```python
from build123d import *

# Parameters (mm, degrees)
SKETCH_1_R          = 50
EXTRUDE_1_DEPTH     = 20
SKETCH_2_R          = 5.25
CUT_EXTRUDE_1_DEPTH = 20
CUT_EXTRUDE_2_DEPTH = 20
SKETCH_4_R          = 50
SKETCH_4_R_2        = 5.25
EXTRUDE_2_DEPTH     = 20


with BuildPart() as part:
    # 草图1 → 凸台-拉伸1 (new body)
    with BuildSketch(Plane(origin=(0, 0, 0), x_dir=(1, 0, 0), z_dir=(0, 1, 0))):
        with Locations(Location((0, 0, 0), (0, 0, 270))):
            Circle(SKETCH_1_R)
    extrude(amount=EXTRUDE_1_DEPTH)

    # 草图2 → 切除-拉伸1 (cut)
    with BuildSketch(Plane(origin=(0, 20, 0), x_dir=(1, 0, 0), z_dir=(0, 1, 0))):
        with Locations(Location((0, 0, 0), (0, 0, 270))):
            Circle(SKETCH_2_R)
    extrude(amount=-CUT_EXTRUDE_1_DEPTH, mode=Mode.SUBTRACT)

    # 草图3 → 切除-拉伸2 (cut)
    with BuildSketch(Plane(origin=(0, 20, 0), x_dir=(1, 0, 0), z_dir=(0, 1, 0))):
        with BuildLine():
            ThreePointArc((42.5, 0), (35, 7.5), (27.5, 0))
            ThreePointArc((27.5, 0), (25.406687144, -10.52379439), (19.445436483, -19.445436483))
            ThreePointArc((19.445436483, -19.445436483), (19.445436477, -30.052038195), (30.052038189, -30.052038212))
            ThreePointArc((30.052038189, -30.052038212), (39.264880129, -16.264045883), (42.5, 0))
        make_face()
        with BuildLine():
            ThreePointArc((2e-09, 27.5), (10.523794391, 25.406687144), (19.445436483, 19.445436483))
            ThreePointArc((19.445436483, 19.445436483), (30.0520382, 19.445436483), (30.0520382, 30.0520382))
            ThreePointArc((30.0520382, 30.0520382), (16.264045902, 39.264880121), (5.8e-08, 42.5))
            ThreePointArc((5.8e-08, 42.5), (-7.5, 35.000000028), (2e-09, 27.5))
        make_face()
        with BuildLine():
            ThreePointArc((-30.0520382, -30.0520382), (-16.264045799, -39.264880163), (1.65e-07, -42.5))
            ThreePointArc((1.65e-07, -42.5), (7.5, -34.999999948), (6.1e-08, -27.5))
            ThreePointArc((6.1e-08, -27.5), (-10.523794348, -25.406687162), (-19.44543646, -19.445436505))
            ThreePointArc((-19.44543646, -19.445436505), (-30.052038189, -19.445436472), (-30.0520382, -30.0520382))
        make_face()
        with BuildLine():
            ThreePointArc((-27.5, 0), (-25.406687154, 10.523794365), (-19.445436521, 19.445436445))
            ThreePointArc((-19.445436521, 19.445436445), (-19.445436492, 30.05203821), (-30.052038258, 30.052038143))
            ThreePointArc((-30.052038258, 30.052038143), (-39.264880164, 16.264045797), (-42.5, -8.9e-08))
            ThreePointArc((-42.5, -8.9e-08), (-34.999999956, -7.5), (-27.5, 0))
        make_face()
    extrude(amount=-CUT_EXTRUDE_2_DEPTH, mode=Mode.SUBTRACT)

    # 草图4 → 凸台-拉伸2 (add)
    # profile 1 of 6: a face of its own
    with BuildSketch(Plane.XZ):
        with Locations(Location((0, 0, 0), (0, 0, 270))):
            Circle(SKETCH_4_R)
        with BuildLine():
            ThreePointArc((30.0520382, 30.0520382), (39.264880132, 16.264045876), (42.5, 0))
            ThreePointArc((42.5, 0), (39.264880132, -16.264045876), (30.0520382, -30.0520382))
            ThreePointArc((30.0520382, -30.0520382), (16.264045876, -39.264880132), (0, -42.5))
            ThreePointArc((0, -42.5), (-16.264045876, -39.264880132), (-30.0520382, -30.0520382))
            ThreePointArc((-30.0520382, -30.0520382), (-39.264880132, -16.264045876), (-42.5, 0))
            ThreePointArc((-42.5, 0), (-39.264880132, 16.264045876), (-30.0520382, 30.0520382))
            ThreePointArc((-30.0520382, 30.0520382), (-16.264045876, 39.264880132), (0, 42.5))
            ThreePointArc((0, 42.5), (16.264045876, 39.264880132), (30.0520382, 30.0520382))
        make_face(mode=Mode.SUBTRACT)
    # profile 2 of 6: a face of its own
    with BuildSketch(Plane.XZ):
        with BuildLine():
            ThreePointArc((0, -42.5), (-7.5, -35), (0, -27.5))
            ThreePointArc((0, -27.5), (-10.52379439, -25.406687144), (-19.445436483, -19.445436483))
            ThreePointArc((-19.445436483, -19.445436483), (-19.445436483, -30.0520382), (-30.0520382, -30.0520382))
            ThreePointArc((-30.0520382, -30.0520382), (-16.264045876, -39.264880132), (0, -42.5))
        make_face()
    # profile 3 of 6: a face of its own
    with BuildSketch(Plane.XZ):
        with BuildLine():
            ThreePointArc((-27.5, 0), (-25.406687144, 10.52379439), (-19.445436483, 19.445436483))
            ThreePointArc((-19.445436483, 19.445436483), (-30.0520382, 19.445436483), (-30.0520382, 30.0520382))
            ThreePointArc((-30.0520382, 30.0520382), (-39.264880132, 16.264045876), (-42.5, 0))
            ThreePointArc((-42.5, 0), (-35, 7.5), (-27.5, 0))
        make_face()
    # profile 4 of 6: a face of its own
    with BuildSketch(Plane.XZ):
        with BuildLine():
            ThreePointArc((0, 27.5), (10.52379439, 25.406687144), (19.445436483, 19.445436483))
            ThreePointArc((19.445436483, 19.445436483), (19.445436483, 30.0520382), (30.0520382, 30.0520382))
            ThreePointArc((30.0520382, 30.0520382), (16.264045876, 39.264880132), (0, 42.5))
            ThreePointArc((0, 42.5), (7.5, 35), (0, 27.5))
        make_face()
    # profile 5 of 6: a face of its own
    with BuildSketch(Plane.XZ):
        with BuildLine():
            ThreePointArc((19.445436483, -19.445436483), (25.406687144, -10.52379439), (27.5, 0))
            ThreePointArc((27.5, 0), (25.406687144, 10.52379439), (19.445436483, 19.445436483))
            ThreePointArc((19.445436483, 19.445436483), (10.52379439, 25.406687144), (0, 27.5))
            ThreePointArc((0, 27.5), (-10.52379439, 25.406687144), (-19.445436483, 19.445436483))
            ThreePointArc((-19.445436483, 19.445436483), (-25.406687144, 10.52379439), (-27.5, 0))
            ThreePointArc((-27.5, 0), (-25.406687144, -10.52379439), (-19.445436483, -19.445436483))
            ThreePointArc((-19.445436483, -19.445436483), (-10.52379439, -25.406687144), (0, -27.5))
            ThreePointArc((0, -27.5), (10.52379439, -25.406687144), (19.445436483, -19.445436483))
        make_face()
        with Locations(Location((0, 0, 0), (0, 0, 90))):
            Circle(SKETCH_4_R_2, mode=Mode.SUBTRACT)
    # profile 6 of 6: a face of its own
    with BuildSketch(Plane.XZ):
        with BuildLine():
            ThreePointArc((42.5, 0), (35, -7.5), (27.5, 0))
            ThreePointArc((27.5, 0), (25.406687144, -10.52379439), (19.445436483, -19.445436483))
            ThreePointArc((19.445436483, -19.445436483), (30.0520382, -19.445436483), (30.0520382, -30.0520382))
            ThreePointArc((30.0520382, -30.0520382), (39.264880132, -16.264045876), (42.5, 0))
        make_face()
    extrude(amount=EXTRUDE_2_DEPTH)


solid = part.part
```
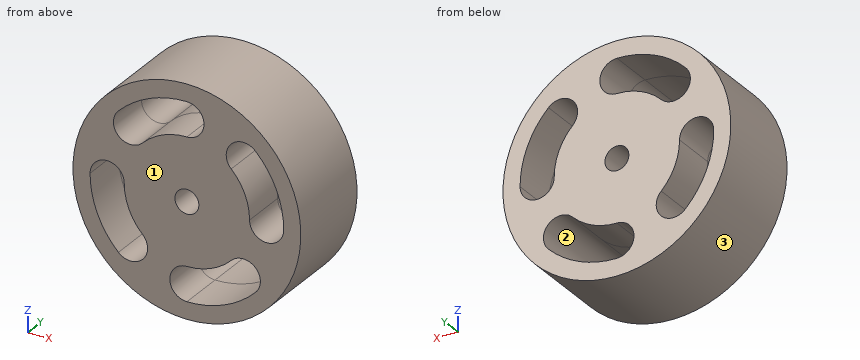
CAD build for the part. Positions are in the model's coordinates, mm. Face numbers are marked on the shaded views. Coordinates: 2 decimals unless noted, no trailing zeros. Order: outer loops, then holes, each group sorted by start corner. A loop starts at its lowest first (then second) coordinate and runs counter-clockwise, first axis right, second up. Notation, with made-up numbers: M 48,22 L 62,22 A26 ccw 62,48 Z; hole C 12,84.25 d7. An arc over 180 degrees is marked long. Write each question's results on one line, items separated by ' | '. Start each with the question number.
Q1. Cut at A-A (y = -11.5). List the corners of the cut face in (x, z).
Q2. Pull direction Z, two halves, no side cores. Call the marked faces 1, 2 and 3: +Z half, -Z half, draft (parallel to the pull), parting line (faces both ways), or undercut.
Q3. Drill centre lines: probe 1 along X at (y, z) = (-11, -19.5); probe 2 along Z at (x, y) = (-19, -1); probe 3 along Z at (x, y) = (-1, 0.5). Where is each one in solid material? Low to high. Write a range as from..to.
Q4. Cut at D-D (x = -23). List the corners of the cut face in (y, z), then the cut area to 3 significant figures.
Q5. Cut at C-C (z = -35). List the corners of the cut face in (x, y).
Q6. Flat gauge pins, fed straight in: P1, Ø5, axis at y = 9.5, z = -39, coming from the -X side; P2, Ø3, axis at x = 3, y = -0.5, coming from the -Z side; P3, Ø1, axis at x = 28, y = 3, coming from the -Z side. Where does each tip first touch, or does it go through?
Q7. Cut at B-B (x = -40). List the corners of the cut face in (y, z), then the cut area to 3 significant figures.
Found:
1) outline: C 0,0 d100; hole M -42.5,0 A42.5 ccw -30.05,-30.05 A7.5 ccw -19.45,-19.45 A27.5 cw -27.5,0 A7.5 ccw Z; hole M -30.05,30.05 A7.5 ccw -19.45,19.45 A27.5 cw 0,27.5 A7.5 ccw 0,42.5 A42.5 ccw Z; hole C 0,0 d10.5; hole M 0,-42.5 A42.5 ccw 30.05,-30.05 A7.5 ccw 19.45,-19.45 A27.5 cw 0,-27.5 A7.5 ccw Z; hole M 19.45,19.45 A27.5 cw 27.5,0 A7.5 ccw 42.5,0 A42.5 ccw 30.05,30.05 A7.5 ccw Z
2) face 1: draft | face 2: undercut | face 3: parting line
3) probe 1: -46.04..-37.76, -19.39..19.39, 30.11..46.04 | probe 2: -46.25..-29.57, -19.93..19.88, 38.02..46.25 | probe 3: -49.99..-42.43, -27.57..-5.15, 5.15..27.48, 42.49..49.99
4) outline: M -20,-44.4 L 20,-44.4 L 20,-32.04 L -20,-32.04 Z; M -20,-15.07 L 20,-15.07 L 20,17.46 L -20,17.46 Z; M -20,35.74 L 20,35.74 L 20,44.4 L -20,44.4 Z | area: 2,140 mm²
5) outline: M -35.71,-20 L -7.5,-20 L -7.5,20 L -35.71,20 Z; M 24.11,-20 L 35.71,-20 L 35.71,20 L 24.11,20 Z
6) P1: x = -34.17 | P2: z = -49.98 | P3: z = -41.76
7) outline: M -20,-30 L 20,-30 L 20,-14.36 L -20,-14.36 Z; M -20,5.59 L 20,5.59 L 20,30 L -20,30 Z | area: 1,600 mm²
